For this review, take the finished solid that the model builds, in its own axes (mm). Round coordinates to 2 decimals unless told otherwise and drop trailing zeros. Put each result on its own line as item: value.
from build123d import *

# Parameters (mm, degrees)
SKETCH1_W           = 76.495
SKETCH1_H           = 6.35
SKETCH1_R           = 1.5875
SKETCH1_W_2         = 63.5
SKETCH1_W_3         = 25.4
BOSS_EXTRUDE1_DEPTH = 3.175


with BuildPart() as part:
    # Sketch1 → Boss-Extrude1 (new body)
    with BuildSketch(Plane(origin=(0, 0, 0), x_dir=(0, 0, -1), z_dir=(1, 0, 0))):
        with Locations((-38.2475, 3.175)):
            Rectangle(SKETCH1_W, SKETCH1_H)
        with Locations((-70.145, 3.175)):
            Circle(SKETCH1_R, mode=Mode.SUBTRACT)
        with Locations((-63.795, 3.175)):
            Circle(SKETCH1_R, mode=Mode.SUBTRACT)
        with Locations((-57.445, 3.175)):
            Circle(SKETCH1_R, mode=Mode.SUBTRACT)
        with Locations((-51.095, 3.175)):
            Circle(SKETCH1_R, mode=Mode.SUBTRACT)
        with Locations((-44.745, 3.175)):
            Circle(SKETCH1_R, mode=Mode.SUBTRACT)
        with Locations((-38.395, 3.175)):
            Circle(SKETCH1_R, mode=Mode.SUBTRACT)
        with Locations((31.75, 3.175)):
            Rectangle(SKETCH1_W_2, SKETCH1_H)
        with Locations((3.175, 3.175)):
            Circle(SKETCH1_R, mode=Mode.SUBTRACT)
        with Locations((60.325, 3.175)):
            Circle(SKETCH1_R, mode=Mode.SUBTRACT)
        with Locations((76.2, 3.175)):
            Rectangle(SKETCH1_W_3, SKETCH1_H)
    extrude(amount=BOSS_EXTRUDE1_DEPTH)


solid = part.part
(1) Add section A-A on x = 1.65. State how many separate pieces and enclosed holes the cut face has, then the cut area to 3 significant figures.
A:
separate pieces: 1
enclosed holes: 8
area: 987 mm2
(2) To check wall thickness, follow L1, parallel to Y at x = 1.8, z = 52. State the ranges of the line that lie inside material, in increasing order.
A:
L1: y = 0 to 1.87, 4.48 to 6.35
(3) Draft analysis for pull direction Y (two halves, no side actions). For faces 1 (the face through (1.57, 3.65, -61.84)), 2 (the face through (2, 3, 76.495)), 3 (the face through (2, 0, -5)), state which applies: released by +Y, released by -Y, zero draft, split by the parting line, or undercut.
A:
face 1: undercut
face 2: zero draft
face 3: released by -Y
